Check sheet for the modelled part. Datum: model origin and axes. Units: mm. Face numbers are marked on the shaded views. A direction names the side the tool comes from. Coordinates: 2 decimals unless noted, no trailing zeros. Write each loop counter-clockwise with the first axis right and the second up, starting at its lowest first coordinate (ties: lowest second). Pieces come first, ordered by that corner, then holes. Notation, with made-up numbers: (27.5, 40.25) -> (37.5, 40.25) arc R28 cw to (37.5, 67.25) -> close; hole circle Ø5 at (3, 44). An arc over 180 degrees is marked (long way). Put each result on its own line as item: value.
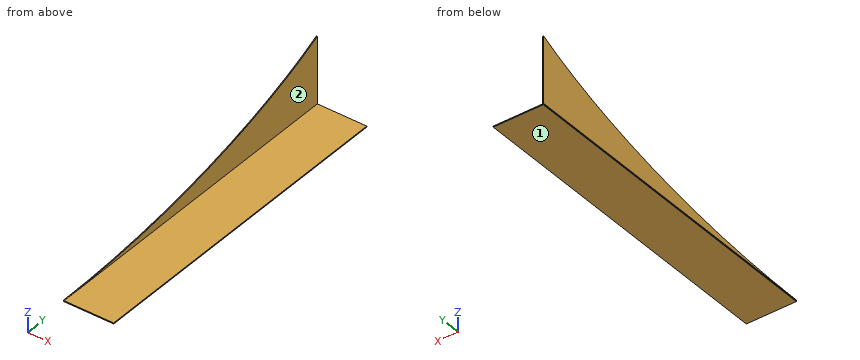
```python
from build123d import *

# Parameters (mm, degrees)
F1_DEPTH = 1.5
F2_E1_W  = 1000
F2_E1_H  = 150
F3_DEPTH = 3


with BuildPart() as f1:
    # F0 (on Right) → F1 (new body, symmetric)
    with BuildSketch(Plane.YZ):
        with BuildLine():
            add(Edge.make_bspline(
                [(-507.5750658325, -64.4556317002), (-152.691480371, -64.4556317002), (239.9747440193, 9.7828772396), (492.4249341675, 135.5443682998)],
                knots=[0, 0, 0, 0, 1019.8039027186, 1019.8039027186, 1019.8039027186, 1019.8039027186], degree=3))
            Line((-507.5750658325, -64.4556317002), (492.4249341675, -64.4556317002))
            Line((492.4249341675, -64.4556317002), (492.4249341675, 135.5443682998))
        make_face()
    extrude(amount=F1_DEPTH, both=True)

    # F2_E1 (on explicit) → F3 (join)
    with BuildSketch(Plane(origin=(0, -507.5750658325, -64.4556317002), x_dir=(0, 1, 0), z_dir=(0, 0, -1))):
        with Locations((500, 75)):
            Rectangle(F2_E1_W, F2_E1_H)
    extrude(amount=F3_DEPTH)


solid = f1.part
```
Q1. Tool access check on the marked faces 1 and 2. Record the directions out of +Z, -Z, +X, -X, +Y, -Y that give a thin tool (end or side, any length) a straight path to the whole face; none if there is none.
Recorded:
face 1: -Z, +X, -X, +Y, -Y
face 2: +Z, +X, +Y, -Y
Q2. Material ranges on line 1 along Z through (x, y) = (74, 343); line 2 along X through (y, z) = (372, 1.5), recorded low to high.
Recorded:
line 1: z = -67.46 to -64.46
line 2: x = -1.5 to 1.5
Q3. Depth check by flat-ended pin: P1, Ø1.5, axis at x = 31.5, y = 392, coming from the +Z side; P2, Ø1.5, axis at y = 171.5, z = -66, coming from the -X side. Enter the tip coordinate at first touch or a pass-through.
Recorded:
P1: stops at z = -64.46
P2: stops at x = 0
Q4. Cross-section at A-A (x = 107.5). Record the cut outline in (y, z), plus the area to 3 significant figures.
Recorded:
outline: (-507.58, -67.46) -> (492.42, -67.46) -> (492.42, -64.46) -> (-507.58, -64.46) -> close
area: 3,000 mm2
